Source: CAD feature listing. Evaluate the final solid. Frame: model axes, mm. Face numbers are marked on the shaded views. A direction names the side the tool comes from. Give positions to 0.01 mm unless a question says otherwise; leave off trailing zeros. Order: outer loops, then holes, each group sorted by start corner. A loop starts at its lowest first (then second) coordinate and runs counter-clockwise, first axis right, second up.
from build123d import *

# Parameters (mm, degrees)
F0_W     = 34.925
F0_H     = 50.8
F0_R     = 1.8288
F0_W_2   = 9.525
F0_H_2   = 12.954
F0_W_3   = 15.875
F0_R_2   = 1.5875
F1_DEPTH = 6.35
F2_D     = 3.6576
F3_D     = 3.7973


with BuildPart() as f1:
    # F0 (on Top) → F1 (new body)
    with BuildSketch(Plane.XY):
        with Locations((-87.3125, 0)):
            Rectangle(F0_W, F0_H)
        with Locations((-100.0125, -20.6375)):
            Circle(F0_R, mode=Mode.SUBTRACT)
        with Locations((-87.3125, -12.573)):
            Rectangle(F0_W_2, F0_H_2, mode=Mode.SUBTRACT)
        with Locations((-74.6125, -20.6375)):
            Circle(F0_R, mode=Mode.SUBTRACT)
        with Locations((-87.3125, 12.573)):
            Rectangle(F0_W_2, F0_H_2, mode=Mode.SUBTRACT)
        with Locations((-100.0125, 20.6375)):
            Circle(F0_R, mode=Mode.SUBTRACT)
        with Locations((-74.6125, 20.6375)):
            Circle(F0_R, mode=Mode.SUBTRACT)
        with Locations((-61.9125, 0)):
            Rectangle(F0_W_3, F0_H)
        with Locations((-61.1378, -15.875)):
            Circle(F0_R_2, mode=Mode.SUBTRACT)
        with Locations((-61.1378, 15.875)):
            Circle(F0_R_2, mode=Mode.SUBTRACT)
        with Locations((-100.0125, -20.6375)):
            Circle(F0_R)
        with Locations((-100.0125, 20.6375)):
            Circle(F0_R)
        with Locations((-74.6125, 20.6375)):
            Circle(F0_R)
        with Locations((-74.6125, -20.6375)):
            Circle(F0_R)
        with Locations((-61.1378, 15.875)):
            Circle(F0_R_2)
        with Locations((-61.1378, -15.875)):
            Circle(F0_R_2)
    extrude(amount=F1_DEPTH)

    # F2 (through all)
    with Locations(Plane(origin=(0, 0, 0), x_dir=(1, 0, 0), z_dir=(0, 0, -1))):
        with Locations((-100.0125, -20.6375), (-74.6125, -20.6375), (-74.6125, 20.6375), (-100.0125, 20.6375)):
            Hole(F2_D / 2)

    # F3 (through all)
    with Locations(Plane(origin=(0, 0, 0), x_dir=(1, 0, 0), z_dir=(0, 0, -1))):
        with Locations((-61.1378, 15.875), (-61.1378, -15.875)):
            Hole(F3_D / 2)


solid = f1.part
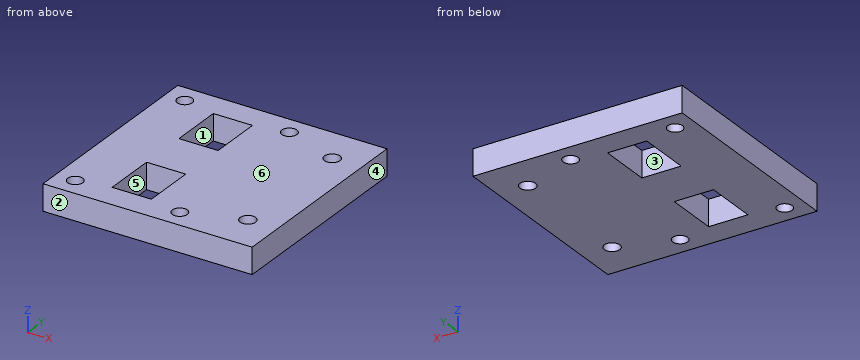
1) Section query A-A on x = -88.5. Output: boundary loops of the cut face in (y, z).
Checks:
outline: (-25.4, 0) - (-19.05, 0) - (-19.05, 6.35) - (-25.4, 6.35) - close; (-6.1, 0) - (6.1, 0) - (6.1, 6.35) - (-6.1, 6.35) - close; (19.05, 0) - (25.4, 0) - (25.4, 6.35) - (19.05, 6.35) - close
2) First-contact query: pin 1 Ø3.5 at (x, y) = (-74.61, -20.64) entering from +Z; pin 2 Ø1 at (x, y) = (-73, -14.5) entering from -Z. Flat tips, straight axial feed; report the tip coordinate or a pass-through.
Checks:
pin 1: passes through
pin 2: stops at z = 0
3) Reachability of the marked faces 5 and 6 from +Z, -Z, +X, -X, +Y, -Y: full face, straight path, thin tool, end or side. Return the list, or none.
Checks:
face 5: +Z, -Z
face 6: +Z, +X, -X, +Y, -Y
4) Section query C-C on z = 2.5. State how many separate pieces and enclosed holes the cut face has, and give its area (3 significant figures).
Checks:
separate pieces: 1
enclosed holes: 8
area: 2,270 mm2
5) Ray query, L1, parallel to Y at x = -84, z = 4.5; L2, parallel to X at y = -20.5, z = 4.5 (3 decimals); L3, parallel to X at y = -7.5, z = 4 (3 decimals). Return the intervals inside material, ascending.
Checks:
L1: y = -25.4 to -19.05, -6.1 to 6.1, 19.05 to 25.4
L2: x = -104.775 to -101.836, -98.189 to -76.436, -72.789 to -53.975
L3: x = -104.775 to -92.075, -82.55 to -53.975
6) Section query B-B on y = -8. Output: boundary loops of the cut face in (x, z) (3 decimals), and give its area (3 significant figures).
Checks:
outline: (-104.775, 0) - (-92.075, 0) - (-92.075, 6.35) - (-104.775, 6.35) - close; (-82.55, 0) - (-53.975, 0) - (-53.975, 6.35) - (-82.55, 6.35) - close
area: 262 mm2
7) Section query D-D on x = -101. Output: boundary loops of the cut face in (y, z), and give its area (3 significant figures).
Checks:
outline: (-25.4, 0) - (-22.18, 0) - (-22.18, 6.35) - (-25.4, 6.35) - close; (-19.1, 0) - (19.1, 0) - (19.1, 6.35) - (-19.1, 6.35) - close; (22.18, 0) - (25.4, 0) - (25.4, 6.35) - (22.18, 6.35) - close
area: 283 mm2
8) Pull-direction query (X, two-part tool) for the marked faces 1, 2, 3 and 4; classes: +X half, -X half, draft (parallel to the pull), parting line (faces both ways), or undercut.
Checks:
face 1: undercut
face 2: draft
face 3: undercut
face 4: +X half
